Geometry: final body of the model. Coordinates: model frame, mm. Face numbers are marked on the shaded views. Round coordinates to 2 decimals unless told otherwise and drop trailing zeros. Loops run counter-clockwise (first coordinate to the right, second up) from the corner with the lowest first, then second, coordinate; pieces in that order, holes last. Notation, with made-up numbers: (-26, 79.25) -> (-22, 79.25) arc R12 ccw to (-22, 84.25) -> close; hole circle Ø3 at (-11.5, 5). An arc over 180 degrees is marked (long way). Answer in a Markdown table with one row per item.
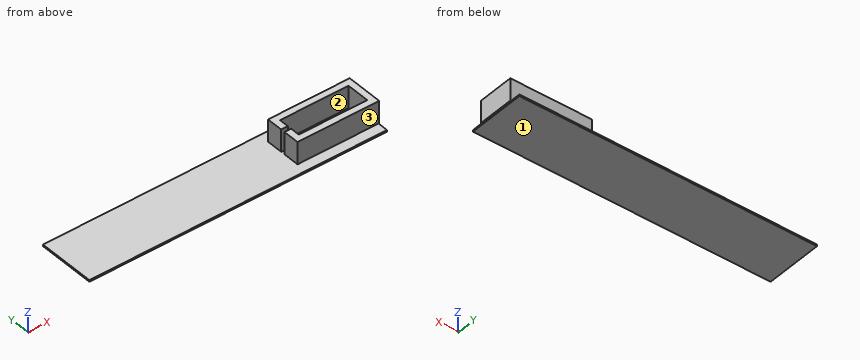
```python
from build123d import *

# Parameters (mm, degrees)
PAD_DEPTH    = 6.7
SKETCH001_W  = 90
SKETCH001_H  = 17.3
PAD001_DEPTH = 0.5


with BuildPart() as part:
    # Sketch (on Sketch) → Pad (new body)
    with BuildSketch(Plane.XY):
        Polygon((-10.35, 3.5), (10.35, 3.5), (10.35, -3.5), (-10.35, -3.5), (-10.35, -0.6), (-12.35, -0.6), (-12.35, -5.5), (12.35, -5.5), (12.35, 5.5), (-12.35, 5.5), (-12.35, 0.6), (-10.35, 0.6), align=None)
    extrude(amount=PAD_DEPTH)

    # Sketch001 → Pad001 (join)
    with BuildSketch(Plane.XY):
        with Locations((-32.851308, 0)):
            Rectangle(SKETCH001_W, SKETCH001_H)
    extrude(amount=-PAD001_DEPTH)


solid = part.part
```
Item 1: Cut plane B-B (y = 1.5). Output: boundary loops of the cut face in (x, z), then the cut area to 3 significant figures.
Answer:
| item | result |
|---|---|
| outline | (-77.85, -0.5) -> (12.15, -0.5) -> (12.15, 0) -> (12.35, 0) -> (12.35, 6.7) -> (10.35, 6.7) -> (10.35, 0) -> (-10.35, 0) -> (-10.35, 6.7) -> (-12.35, 6.7) -> (-12.35, 0) -> (-77.85, 0) -> close |
| area | 71.8 mm² |
Item 2: Cut plane C-C (x = -20). Output: boundary loops of the cut face in (y, z), then the cut area to 3 significant figures.
Answer:
| item | result |
|---|---|
| outline | (-8.65, -0.5) -> (8.65, -0.5) -> (8.65, 0) -> (-8.65, 0) -> close |
| area | 8.65 mm² |
Item 3: Draft query along Y for the marked faces 1, 2 and 3. Return one class per face: pulls with the +Y half, pulls with the -Y half, needs draft (parallel to the pull), parting line crosses it, or undercut.
Answer:
| item | result |
|---|---|
| face 1 | needs draft |
| face 2 | undercut |
| face 3 | pulls with the -Y half |
Item 4: Line query: probe 1 along X at (y, z) = (2.5, 0.75); probe 2 along Y at (x, z) = (-4, 1.5); probe 3 along X at (y, z) = (-0.5, 4.5). Output: solid intervals per line, ascending. Write a range as [from, to].
Answer:
| item | result |
|---|---|
| probe 1 | x = [-12.35, -10.35], [10.35, 12.35] |
| probe 2 | y = [-5.5, -3.5], [3.5, 5.5] |
| probe 3 | x = [10.35, 12.35] |
Item 5: Cut plane A-A (z = 2.25). Output: boundary loops of the cut face in (x, y).
Answer:
| item | result |
|---|---|
| outline | (-12.35, -5.5) -> (12.35, -5.5) -> (12.35, 5.5) -> (-12.35, 5.5) -> (-12.35, 0.6) -> (-10.35, 0.6) -> (-10.35, 3.5) -> (10.35, 3.5) -> (10.35, -3.5) -> (-10.35, -3.5) -> (-10.35, -0.6) -> (-12.35, -0.6) -> close |
Item 6: Cut plane D-D (y = -6.75). Output: boundary loops of the cut face in (x, z), then the cut area to 3 significant figures.
Answer:
| item | result |
|---|---|
| outline | (-77.85, -0.5) -> (12.15, -0.5) -> (12.15, 0) -> (-77.85, 0) -> close |
| area | 45.0 mm² |
Item 7: Pin query (flat end, axial travel): pin 1 Ø2 at (x, z) = (1, 4) entering from -Y; pin 2 Ø1.5 at (y, z) = (2.5, 3) entering from -X; pin 3 Ø3.5 at (x, z) = (2, 3.5) entering from +Y. Return the tip coordinate at first contact, or that it passes through.
Answer:
| item | result |
|---|---|
| pin 1 | stops at y = -5.5 |
| pin 2 | stops at x = -12.35 |
| pin 3 | stops at y = 5.5 |
